The model under review builds one solid part; all positions refer to its coordinate system, in mm. A direction names the side the tool comes from. Give positions to 0.01 mm unless a question says otherwise; leave off trailing zeros. Loops run counter-clockwise (first coordinate to the right, second up) from the corner with the lowest first, then second, coordinate; pieces in that order, holes last. Notation, with made-up numbers: (15, -5) - (73, -5) arc R24 ccw to (73, 10) - close; hole circle Ø3 at (-4.5, 88). An arc over 180 degrees is marked (long way). Return JSON: item names as keys, results as strings. Group by question number.
from build123d import *

# Parameters (mm, degrees)
BOSS_EXTRUDE1_DEPTH     = 0.9
SKETCH8_R               = 3
SKETCH8_R_2             = 2.5
BOSS_EXTRUDE2_DEPTH     = 1.2
CUT_EXTRUDE1_DEPTH      = 11.070253224
CUT_EXTRUDE1_DEPTH_BACK = 11.070253224
SKETCH1_R               = 2.5
SWEEP1_PITCH            = 0.8
SPLIT1_START            = -3.0000001
SPLIT1_OUTLINE_W        = 8
SPLIT1_OUTLINE_H        = 2.1
SPLIT1_OUTLINE_H_2      = 1.9
SPLIT1_DEPTH            = 6.0000002


with BuildPart() as part:
    # Sketch7 → Boss-Extrude1 (new, symmetric)
    with BuildSketch(Plane.XY):
        with BuildLine():
            Line((-7.92820323, 4), (4.92820323, 4))
            ThreePointArc((4.92820323, 4), (6, 0), (4.92820323, -4))
            Line((4.92820323, -4), (-7.92820323, -4))
            ThreePointArc((-7.92820323, -4), (-9, 0), (-7.92820323, 4))
        make_face()
    extrude(amount=BOSS_EXTRUDE1_DEPTH, both=True)

    # Sketch8 → Boss-Extrude2 (add)
    with BuildSketch(Plane.XY.offset(0.9)):
        with Locations(Location((0, 0, 0), (0, 0, 180))):
            Circle(SKETCH8_R)
        Circle(SKETCH8_R_2, mode=Mode.SUBTRACT)
    extrude(amount=BOSS_EXTRUDE2_DEPTH)

    # Sketch1 → Cut-Extrude1 (cut, two sides: drawn at the far end of the back side and taken through both)
    with BuildSketch(Plane.XY.offset(-CUT_EXTRUDE1_DEPTH_BACK)):
        Circle(SKETCH1_R)
    extrude(amount=CUT_EXTRUDE1_DEPTH + CUT_EXTRUDE1_DEPTH_BACK, mode=Mode.SUBTRACT)

    # Sweep1: arcs per turn and ends read off the stored shape
    # Sweep1: the profile of Sketch3 screwed along a right-hand helix through 4.75 turns, 8 arcs to a turn; built about Z, then put on its axis
    sweep1_z = Axis((0, 0, 0), (0, 0, 1))
    sweep1_corners = [(2.54330127, 0, 0.025), (2.54330127, 0, -0.725), (1.980384758, 0, -0.4), (1.980384758, 0, -0.3)]
    with BuildLine(mode=Mode.PRIVATE) as sweep1_profile:
        Line(sweep1_corners[0], sweep1_corners[1])
        Line(sweep1_corners[1], sweep1_corners[2])
        Line(sweep1_corners[2], sweep1_corners[3])
        Line(sweep1_corners[3], sweep1_corners[0])
    sweep1_cap = Face(sweep1_profile.wire())
    sweep1_turn_angles = [0, 22.5, 45, 67.5, 90, 112.5, 135, 157.5, 180, 202.5, 225, 247.5, 270, 292.5, 315, 337.5, 360]
    sweep1_turn_weights = [1, 0.9238795325112867, 1, 0.9238795325112867, 1, 0.9238795325112867, 1, 0.9238795325112867, 1, 0.9238795325112867, 1, 0.9238795325112867, 1, 0.9238795325112867, 1, 0.9238795325112867, 1]
    sweep1_turn_rails = [Edge.make_bspline([Vector(p[0], p[1], 0).rotate(sweep1_z, sweep1_turn_angles[k]) / sweep1_turn_weights[k] + Vector(0, 0, p[2] + SWEEP1_PITCH * sweep1_turn_angles[k] / 360) for k in range(17)], [0, 0, 0, 1, 1, 2, 2, 3, 3, 4, 4, 5, 5, 6, 6, 7, 7, 8, 8, 8], 2, sweep1_turn_weights) for p in sweep1_corners]
    sweep1_turn_sides = [Face.make_surface_from_curves(sweep1_turn_rails[p[0]], sweep1_turn_rails[p[1]]) for p in [(0, 1), (1, 2), (2, 3), (3, 0)]]
    sweep1_last_angles = [1440, 1462.5, 1485, 1507.5, 1530, 1552.5, 1575, 1597.5, 1620, 1642.5, 1665, 1687.5, 1710]
    sweep1_last_weights = [1, 0.9238795325112867, 1, 0.9238795325112867, 1, 0.9238795325112867, 1, 0.9238795325112867, 1, 0.9238795325112867, 1, 0.9238795325112776, 1]
    sweep1_last_rails = [Edge.make_bspline([Vector(p[0], p[1], 0).rotate(sweep1_z, sweep1_last_angles[k]) / sweep1_last_weights[k] + Vector(0, 0, p[2] + SWEEP1_PITCH * sweep1_last_angles[k] / 360) for k in range(13)], [0, 0, 0, 1, 1, 2, 2, 3, 3, 4, 4, 5, 5, 6, 6, 6], 2, sweep1_last_weights) for p in sweep1_corners]
    sweep1_last_sides = [Face.make_surface_from_curves(sweep1_last_rails[p[0]], sweep1_last_rails[p[1]]) for p in [(0, 1), (1, 2), (2, 3), (3, 0)]]
    sweep1 = Plane(origin=(0, 0, -0.9), x_dir=(0, 1, 0), z_dir=(0, 0, 1)) * Solid(Shell([*[p.moved(Location((0, 0, SWEEP1_PITCH * i))) for i in range(4) for p in sweep1_turn_sides], *sweep1_last_sides, sweep1_cap, sweep1_cap.rotate(sweep1_z, 1710).moved(Location((0, 0, SWEEP1_PITCH * 1710 / 360)))]))
    add(sweep1)

    # Split1: read off the stored shape, not the designer's step
    # Split1 outline → Split1 (cut)
    with BuildSketch(Plane(origin=(0, 0, 0), x_dir=(1, 0, 0), z_dir=(0, 1, 0)).offset(SPLIT1_START)):
        with Locations((0, 1.95)):
            Rectangle(SPLIT1_OUTLINE_W, SPLIT1_OUTLINE_H)
        with Locations((0, -3.05)):
            Rectangle(SPLIT1_OUTLINE_W, SPLIT1_OUTLINE_H_2)
    extrude(amount=SPLIT1_DEPTH, mode=Mode.SUBTRACT)

    # Cut-Extrude2 cone 1 section (through the dimple's axis) → Cut-Extrude2 (revolve, cut)
    with BuildSketch(Plane(origin=(0, 0, -0.9), x_dir=(0, 1, 0), z_dir=(1, 0, 0))):
        Polygon((0, 0), (2.5, 0), (0, 2.5), align=None)
    revolve(axis=Axis((0, 0, -0.9), (0, 0, 1)), mode=Mode.SUBTRACT)

    # Cut-Extrude3 cone 1 section (through the dimple's axis) → Cut-Extrude3 (revolve, cut)
    with BuildSketch(Plane(origin=(0, 0, 2.1), x_dir=(0, -1, 0), z_dir=(1, 0, 0))):
        Polygon((0, 0), (2.5, 0), (0, 2.5), align=None)
    revolve(axis=Axis((0, 0, 2.1), (0, 0, -1)), mode=Mode.SUBTRACT)


solid = part.part
Item 1: Take a section at B-B (x = -6.5). State the section outline as (y, z) points.
Item 2: For L1, parallel to Z at x = -3, y = 1.75; L2, parallel to X at y = 0.25, z = -0.4; L3, parallel to X at y = 1, z = -0.2, list the stretches that pass through material, from the lowest coordinate up. Write a range as from..to.
Item 3: For P1, Ø1.5, axis at y = -2, z = 1.5, coming from the +X side; P2, Ø4.5, axis at x = 0, y = 0, coming from the +Z side; P3, Ø1, axis at x = -2.5, y = -2.5, coming from the +Z side, all flat-tipped, find the tip position at first contact; note any pin that passes through.
Item 4: Tool access review of faces 1 (the face through (6, 0, 0)), 2 (the face through (-2.86, -0.9, 1.49)): name each direction out of +Z, -Z, +X, -X, +Y, -Y from which nothing blocks a thin tool from reaching the whole face with its end or side.
Item 5: Take a section at C-C (y = -3.5). State the section outline as (x, z) points, then the cut area to 3 significant figures.
Item 6: Take a section at A-A (y = 2.75). State the section outline as (x, z) points, then the cut area to 3 significant figures.
Check sheet entries:
{
 "1": {"outline": "(-4, -0.9) - (4, -0.9) - (4, 0.9) - (-4, 0.9) - close"},
 "2": {"L1": "z = -0.9..0.9", "L2": "x = -9..-2.11, 2.29..6", "L3": "x = -8.94..-1.84, 2.29..5.94"},
 "3": {"P1": "stops at x = 5.85", "P2": "stops at z = 1.85", "P3": "stops at z = 0.9"},
 "4": {"face 1": "+Z, -Z, +X", "face 2": "+Z"},
 "5": {"outline": "(-8.19, -0.9) - (5.19, -0.9) - (5.19, 0.9) - (-8.19, 0.9) - close", "area": "24.1 mm^2"},
 "6": {"outline": "(-8.51, -0.9) - (5.51, -0.9) - (5.51, 0.9) - (1.2, 0.9) - (1.2, 2.1) - (-1.2, 2.1) - (-1.2, 0.9) - (-8.51, 0.9) - close", "area": "28.1 mm^2"}
}
